Check sheet for the modelled part. Datum: model origin and axes. Units: mm. A direction names the side the tool comes from. Give positions to 0.01 mm unless a question says otherwise; leave off trailing zeros. Loops run counter-clockwise (first coordinate to the right, second up) from the corner with the lowest first, then second, coordinate; pieces in that order, holes last. Notation, with made-up numbers: (4.25, 24) -> (63.25, 24) arc R4 cw to (63.25, 29) -> close; hole circle Ø3 at (75.25, -21). An arc over 180 degrees is marked (long way). Write each question's results on one line, items separated by ' | '. Start each with the question number.
Item 1: Access from +Z, -Z, +X, -X, +Y, -Y to the whole of each face (thin tool, end or side, straight path). Record for faces 4 (the face through (-4.88, 37.18, 11.42)), 5 (the face through (23.2, -23.2, 0)).
Item 2: Cross-section at B-B on y = 0. Enter the section's corners in (x, z), then the cut area to 3 significant figures.
Item 3: Gauge pin test, flat ends, axial feed: pin 1 Ø8 at (x, z) = (-42.5, 13) entering from -Y; pin 2 Ø6 at (x, y) = (-48.26, 8.51) entering from +Z; pin 3 Ø1.5 at (x, z) = (17.5, 1.5) entering from -Y. Record the tip position at first contact, or that the pin passes through.
Item 4: Cross-section at D-D on z = 4.5. Enter the section's corners in (x, y), then the cut area to 3 significant figures.
Item 5: Scan lines: line 1 along X through (y, z) = (1, 4.75); line 2 along Y through (x, z) = (-9.5, 6.5); line 3 along Z through (x, y) = (46, -15). Record each from-to range of solid material in increasing order.
Item 6: Cross-section at A-A on x = -23.5. Enter the section's corners in (y, z), then the cut area to 3 significant figures.
Item 7: Mould release check, pull along Y, two halves, no side actions. Record for faces 1 (the face through (40.06, 12.62, 9.9)), 2 (the face through (16, -40, 3)), 3 (the face through (-11, 31, 6)): pulls with the +Y half, pulls with the -Y half, needs draft (parallel to the pull), parting line crosses it, or undercut.
Item 8: Cross-section at C-C on x = 0. Enter the section's corners in (y, z).
from build123d import *

# Parameters (mm, degrees)
SKETCH_R      = 54
SKETCH_R_2    = 32.5
SKETCH_R_3    = 2.5
PAD_DEPTH     = 3
SKETCH002_R   = 42
SKETCH002_R_2 = 37.5
PAD002_DEPTH  = 14
SKETCH003_R   = 37.5
SKETCH003_R_2 = 32.5
PAD003_DEPTH  = 3


with BuildPart() as part:
    # Sketch → Pad (new body)
    with BuildSketch(Plane.XY):
        Circle(SKETCH_R)
        Circle(SKETCH_R_2, mode=Mode.SUBTRACT)
        with Locations((0, 49)):
            Circle(SKETCH_R_3, mode=Mode.SUBTRACT)
        with Locations((48.25558, 8.508761)):
            Circle(SKETCH_R_3, mode=Mode.SUBTRACT)
        with Locations((42.435245, -24.5)):
            Circle(SKETCH_R_3, mode=Mode.SUBTRACT)
        with Locations((16.758987, -46.044938)):
            Circle(SKETCH_R_3, mode=Mode.SUBTRACT)
        with Locations((-16.758987, -46.044938)):
            Circle(SKETCH_R_3, mode=Mode.SUBTRACT)
        with Locations((-42.435245, -24.5)):
            Circle(SKETCH_R_3, mode=Mode.SUBTRACT)
        with Locations((-48.25558, 8.508761)):
            Circle(SKETCH_R_3, mode=Mode.SUBTRACT)
        with Locations((-31.496593, 37.536178)):
            Circle(SKETCH_R_3, mode=Mode.SUBTRACT)
        with Locations((31.496593, 37.536178)):
            Circle(SKETCH_R_3, mode=Mode.SUBTRACT)
    extrude(amount=PAD_DEPTH)

    # Sketch002 → Pad002 (join)
    with BuildSketch(Plane.XY.offset(3)):
        Circle(SKETCH002_R)
        Circle(SKETCH002_R_2, mode=Mode.SUBTRACT)
    extrude(amount=PAD002_DEPTH)

    # Sketch003 (on Face15 of Pad002) → Pad003 (join)
    with BuildSketch(Plane.XY.offset(3)):
        Circle(SKETCH003_R)
        Circle(SKETCH003_R_2, mode=Mode.SUBTRACT)
    extrude(amount=PAD003_DEPTH)


solid = part.part
Answer sheet:
1) face 4: +Z | face 5: -Z, +X, -X, +Y, -Y
2) outline: (-54, 0) -> (-32.5, 0) -> (-32.5, 6) -> (-37.5, 6) -> (-37.5, 17) -> (-42, 17) -> (-42, 3) -> (-54, 3) -> close; (32.5, 0) -> (54, 0) -> (54, 3) -> (42, 3) -> (42, 17) -> (37.5, 17) -> (37.5, 6) -> (32.5, 6) -> close | area: 285 mm²
3) pin 1: stops at y = -16.79 | pin 2: stops at z = 3 | pin 3: stops at y = -51.34
4) outline: circle Ø84 at (0, 0); hole circle Ø65 at (0, 0) | area: 2,220 mm²
5) line 1: x = -41.99 to -32.48, 32.48 to 41.99 | line 2: y = -40.91 to -36.28, 36.28 to 40.91 | line 3: z = 0 to 3
6) outline: (-48.62, 0) -> (-22.45, 0) -> (-22.45, 6) -> (-29.22, 6) -> (-29.22, 17) -> (-34.81, 17) -> (-34.81, 3) -> (-48.62, 3) -> close; (22.45, 0) -> (48.62, 0) -> (48.62, 3) -> (34.81, 3) -> (34.81, 17) -> (29.22, 17) -> (29.22, 6) -> (22.45, 6) -> close | area: 354 mm²
7) face 1: parting line crosses it | face 2: needs draft | face 3: undercut
8) outline: (-54, 0) -> (-32.5, 0) -> (-32.5, 6) -> (-37.5, 6) -> (-37.5, 17) -> (-42, 17) -> (-42, 3) -> (-54, 3) -> close; (32.5, 0) -> (46.5, 0) -> (46.5, 3) -> (42, 3) -> (42, 17) -> (37.5, 17) -> (37.5, 6) -> (32.5, 6) -> close; (51.5, 0) -> (54, 0) -> (54, 3) -> (51.5, 3) -> close
